Could you check a few things on this model? Use its own coordinates, in mm. A direction names the side the tool comes from. Give positions to 0.01 mm unless a question says otherwise; leave off trailing zeros. Order: outer loops, then holes, each group sorted by start corner. A loop starts at its lowest first (then second) coordinate and runs counter-clockwise, first axis right, second up.
Autodesk Inventor part; units mm, degrees
ref_plane "lovra_XY" through (12.7, 0, 0) normal (1, 0, 0) x (0, 1, 0)
ref_plane "lovra_YZ" through (12.7, 0, 0) normal (0, 1, 0) x (0, 0, 1)
ref_plane "lovra_ZX" through (12.7, 0, 0) normal (0, 0, 1) x (1, 0, 0)
sketch "Sketch_1" plane through (0, 0, 0) normal (0, 0, 1) x (1, 0, 0)
  line L0 (12.7, 0) -> (0, 0)
  line L1 (0, 0) -> (0, 8.9091)
  line L2 (0, 8.9091) -> (0.762, 9.671)
  line L3 (0.762, 9.671) -> (2.4384, 9.671)
  line L4 (2.4384, 9.671) -> (3.2004, 8.9091)
  line L5 (3.2004, 8.9091) -> (3.9624, 8.9091)
  line L6 (3.9624, 8.9091) -> (3.9624, 10.2235)
  line L7 (3.9624, 10.2235) -> (12.7, 10.2235)
  line L8 (12.7, 10.2235) -> (12.7, 0)
  line L9 (12.7, 0) -> (0, 0)
revolve "Revolution1" add sketch "Sketch_1" angle 360 about axis through (12.7, 0, 0) along (1, 0, 0)
sketch "Sketch_24" plane through (0, 0, 0) normal (0, 0, 1) x (1, 0, 0)
  line L0 (3.9624, 0) -> (3.2004, 0)
  line L1 (3.0477, 10.2235) -> (3.0477, 10.1393)
  line L2 (3.0477, 10.1393) -> (3.8399, 9.3472)
  arc A0 (3.8399, 9.1676) -> (3.8399, 9.3472) centre (3.7501, 9.2574) ccw
  line L3 (3.8399, 9.1676) -> (3.5814, 8.9091)
  line L4 (3.5814, 8.9091) -> (3.2004, 8.9091)
  line L5 (3.2004, 8.9091) -> (3.2004, 8.655)
  line L6 (3.2004, 8.655) -> (3.9624, 8.655)
  line L7 (3.9624, 8.655) -> (3.9624, 9.512)
  line L8 (3.9624, 9.512) -> (3.2509, 10.2235)
  line L9 (3.2509, 10.2235) -> (3.0477, 10.2235)
revolve "Revolution2" add sketch "Sketch_24" angle 360 about axis through (3.9624, 0, 0) along (1, 0, 0)
sketch "Sketch_26" plane through (0, 0, 0) normal (0, 0, 1) x (1, 0, 0)
  line L0 (0, 0) -> (-3.175, 0)
  line L1 (-3.175, 0) -> (-3.175, 6.3754)
  line L2 (-3.175, 6.3754) -> (-2.413, 7.1374)
  line L3 (-2.413, 7.1374) -> (0, 7.1374)
  line L4 (0, 7.1374) -> (0, 0)
  line L5 (0, 0) -> (-3.175, 0)
revolve "Revolution3" add sketch "Sketch_26" angle 360 about axis through (0, 0, 0) along (1, 0, 0)
ref_plane "lovra_XY" through (12.7, 0, 0) normal (1, 0, 0) x (0, 1, 0)
ref_plane "lovra_YZ" through (12.7, 0, 0) normal (0, 1, 0) x (0, 0, 1)
ref_plane "lovra_ZX" through (12.7, 0, 0) normal (0, 0, 1) x (1, 0, 0)
ref_plane "lovra1_XY" through (7.9248, 0, 0) normal (1, 0, 0) x (0, 0, -1)
ref_plane "lovra1_YZ" through (7.9248, 0, 0) normal (0, 0, -1) x (0, 1, 0)
ref_plane "lovra1_ZX" through (7.9248, 0, 0) normal (0, 1, 0) x (1, 0, 0)
ref_plane "lovra2_XY" through (7.9248, 7.874, 0) normal (1, 0, 0) x (0, 0, -1)
ref_plane "lovra2_YZ" through (7.9248, 7.874, 0) normal (0, 0, -1) x (0, 1, 0)
ref_plane "lovra2_ZX" through (7.9248, 7.874, 0) normal (0, 1, 0) x (1, 0, 0)
ref_plane "lovra21_XY" through (0, 0, 5.2705) normal (1, 0, 0) x (0, 0, -1)
ref_plane "lovra21_YZ" through (0, 0, 5.2705) normal (0, 0, -1) x (0, 1, 0)
ref_plane "lovra21_ZX" through (0, 0, 5.2705) normal (0, 1, 0) x (1, 0, 0)
ref_plane "lovra22_XY" through (0, 0, -5.2705) normal (1, 0, 0) x (0, 0, -1)
ref_plane "lovra22_YZ" through (0, 0, -5.2705) normal (0, 0, -1) x (0, 1, 0)
ref_plane "lovra22_ZX" through (0, 0, -5.2705) normal (0, 1, 0) x (1, 0, 0)
ref_plane "lovra3_XY" through (7.9248, -7.874, 0) normal (1, 0, 0) x (0, 0, -1)
ref_plane "lovra3_YZ" through (7.9248, -7.874, 0) normal (0, 0, -1) x (0, 1, 0)
ref_plane "lovra3_ZX" through (7.9248, -7.874, 0) normal (0, 1, 0) x (1, 0, 0)
ref_plane "olen_XY" through (12.7, 0, 0) normal (1, 0, 0) x (0, 0, -1)
ref_plane "olen_YZ" through (12.7, 0, 0) normal (0, 0, -1) x (0, 1, 0)
ref_plane "olen_ZX" through (12.7, 0, 0) normal (0, 1, 0) x (1, 0, 0)
ref_plane "to_mounting_bracket_XY" through (23.0124, 0, 0) normal (1, 0, 0) x (0, 0, -1)
ref_plane "to_mounting_bracket_YZ" through (23.0124, 0, 0) normal (0, 0, -1) x (0, 1, 0)
ref_plane "to_mounting_bracket_ZX" through (23.0124, 0, 0) normal (0, 1, 0) x (1, 0, 0)
ref_plane "to_nut_XY" through (0, 0, 0) normal (1, 0, 0) x (0, 0, -1)
ref_plane "to_nut_YZ" through (0, 0, 0) normal (0, 0, -1) x (0, 1, 0)
ref_plane "to_nut_ZX" through (0, 0, 0) normal (0, 1, 0) x (1, 0, 0)
ref_plane "to_pin_XY" through (33.3248, 0, 0) normal (0, 0, 1) x (1, 0, 0)
ref_plane "to_pin_YZ" through (33.3248, 0, 0) normal (1, 0, 0) x (0, 1, 0)
ref_plane "to_pin_ZX" through (33.3248, 0, 0) normal (0, 1, 0) x (0, 0, 1)
ref_plane "to_screw_XY" through (17.4752, 2.032, -6.0452) normal (0, 1, 0) x (1, 0, 0)
ref_plane "to_screw_YZ" through (17.4752, 2.032, -6.0452) normal (1, 0, 0) x (0, 0, -1)
ref_plane "to_screw_ZX" through (17.4752, 2.032, -6.0452) normal (0, 0, -1) x (0, 1, 0)
ref_plane "to_tube_XY" through (3.2004, 0, 0) normal (1, 0, 0) x (0, 0, -1)
ref_plane "to_tube_YZ" through (3.2004, 0, 0) normal (0, 0, -1) x (0, 1, 0)
ref_plane "to_tube_ZX" through (3.2004, 0, 0) normal (0, 1, 0) x (1, 0, 0)
properties part number "04R0000_rear_head"
Item 1: For pin 1 (6 mm diameter, centred on x = 7, z = -6.5, fed in from +Y); pin 2 (4 mm diameter, centred on x = 1, y = 4, fed in from +Z); pin 3 (1.5 mm diameter, centred on x = -1, z = -5.5, fed in from -Y), each with a flat end and sliding along its axis, tell me the tip position at first contact or that it passes through.
Findings:
pin 1: stops at y = 9.61
pin 2: stops at z = 9.46
pin 3: stops at y = -5.33
Item 2: Please list where these lines run through material, in increasing order: line 1 along X through (y, z) = (-6, 6.25); line 2 along X through (y, z) = (-6.25, -8); line 3 along X through (y, z) = (8.75, 2).
Findings:
line 1: x = 0 to 12.7
line 2: x = 3.05 to 3.32, 3.96 to 12.7
line 3: x = 0.07 to 3.13, 3.65 to 12.7
Item 3: Imagine slicing it at C-C on x = 8.5. List the corners of the cut face in (y, z) for me.
Findings:
outline: circle Ø20.45 at (0, 0)
Item 4: For faces 1 (the cylindrical face through (8.392, -8.113, -6.221)), 2 (the cylindrical face through (1.61, -2.1, -9.44)), 3 (the flat face through (3.962, 7, -7)), which set-ups out of +Z, -Z, +X, -X, +Y, -Y let a thin tool reach every point of the face, with its end or its side?
Findings:
face 1: +X, -X
face 2: -X
face 3: none
Item 5: We'd pull the mould along Y, two halves only. Please class faces 4 (the cylindrical face through (-1.19, -7.13, 0.31)), 5 (the flat face through (-3.175, 0, 0)), 6 (the cylindrical face through (3.394, -1.931, -8.697)): +Y half, -Y half, draft (parallel to the pull), parting line (faces both ways), or undercut.
Findings:
face 4: parting line
face 5: draft
face 6: undercut
